Verification items for the finished model (mm, model axes). A direction names the side the tool comes from. Give positions to 0.01 mm unless a question says otherwise; leave off trailing zeros. Order: outer loops, then holes, each group sorted by start corner. A loop starts at its lowest first (then second) coordinate and runs counter-clockwise, first axis right, second up.
(1) Mould release check, pull along Y, two halves, no side actions. Record for faces 1 (the face through (-6, 17, -3)), 2 (the face through (4.769, 6.493, -21.477)), 3 (the face through (-4.207, -0.077, -18.944)): pulls with the +Y half, pulls with the -Y half, needs draft (parallel to the pull), parting line crosses it, or undercut.
(2) Access from +Z, -Z, +X, -X, +Y, -Y to the whole of each face (thin tool, end or side, straight path). Record for faces 4 (the face through (6, 5, 0)), 5 (the face through (14.985, 11.683, 0.66)), 6 (the face through (-11.25, -5.5, 16.03)).
(3) Sectioned sample at D-D on y = 3.25. Record the cut outline in (x, z) (3 decimals).
(4) Scan lines: L1, parallel to Z at x = 0, y = 9.25; L2, parallel to Y at x = 15, z = 11.5; L3, parallel to Z at x = -4, y = -2.75. Record each from-to range of solid material in increasing order.
(5) Gauge pin test, flat ends, axial feed: pin 1 (4 mm diameter, centred on y = 14, z = 14, fed in from -X); pin 2 (4 mm diameter, centred on y = 5, z = -11, fed in from +X); pin 3 (3 mm diameter, centred on y = -3.5, z = -17, fed in from -X). Record the tip position at first contact, or that the pin passes through.
(6) Sectioned sample at C-C on y = 15.25. Record the cut outline in (x, z), plus the area to 3 significant figures.
```python
from build123d import *

# Parameters (mm, degrees)
F0_R     = 19.405
F1_DEPTH = 5.5
F2_R     = 22
F3_DEPTH = 1.5
F4_R     = 22
F5_DEPTH = 1.5
F6_R     = 15
F7_DEPTH = 10
F8_R     = 6
F9_DEPTH = 24.001
F10_SIZE = 0.5


with BuildPart() as f1:
    # F0 (on Front) → F1 (new body, symmetric)
    with BuildSketch(Plane.XZ):
        Circle(F0_R)
    extrude(amount=F1_DEPTH, both=True)

    # F2 (on face) → F3 (join)
    with BuildSketch(Plane.XZ.offset(5.5)):
        Circle(F2_R)
    extrude(amount=F3_DEPTH)

    # F4 (on face) → F5 (join)
    with BuildSketch(Plane(origin=(0, 5.5, 0), x_dir=(-1, 0, 0), z_dir=(0, 1, 0))):
        Circle(F4_R)
    extrude(amount=F5_DEPTH)

    # F6 (on face) → F7 (join)
    with BuildSketch(Plane(origin=(0, 7, 0), x_dir=(-1, 0, 0), z_dir=(0, 1, 0))):
        Circle(F6_R)
    extrude(amount=F7_DEPTH)

    # F8 (on face) → F9 (cut, through all)
    with BuildSketch(Plane(origin=(0, 17, 0), x_dir=(-1, 0, 0), z_dir=(0, 1, 0))):
        Circle(F8_R)
    extrude(amount=-F9_DEPTH, mode=Mode.SUBTRACT)

    # F10
    f10_edges = [f1.edges().sort_by_distance(p)[0] for p in [
        (6, -7, 0),
        (6, 17, 0),
        (-22, -5.5, 0),
        (22, 5.5, 0),
        (15, 17, 0),
    ]]
    chamfer(f10_edges, length=F10_SIZE)


solid = f1.part
```
Ans:
1. face 1: pulls with the +Y half
1. face 2: needs draft
1. face 3: undercut
2. face 4: +Y, -Y
2. face 5: +Y
2. face 6: none
3. outline: circle Ø38.81 at (0, 0); hole circle Ø12 at (0, 0)
4. L1: z = -15 to -6, 6 to 15
4. L2: y = -7 to 7
4. L3: z = -18.99 to -4.47, 4.47 to 18.99
5. pin 1: stops at x = -9
5. pin 2: stops at x = 19.95
5. pin 3: stops at x = -11.67
6. outline: circle Ø30 at (0, 0); hole circle Ø12 at (0, 0)
6. area: 594 mm2
